Source: CAD feature listing. Evaluate the final solid. Frame: model axes, mm. Round coordinates to 2 decimals unless told otherwise and drop trailing zeros. Write each loop counter-clockwise with the first axis right and the second up, starting at its lowest first coordinate (ties: lowest second). Pieces come first, ordered by that corner, then holes. Notation, with made-up numbers: (35.25, 68.5) -> (44.25, 68.5) arc R17 cw to (44.25, 101.5) -> close; hole circle Ø2 at (25, 81). An arc over 180 degrees is marked (long way). Put each result on its own line as item: value.
```python
from build123d import *

# Parameters (mm, degrees)
F0_W           = 144
F0_H           = 20
F1_DEPTH       = 6
F3_D           = 6.7564
F3_DEPTH       = 16.51
F3_CSINK_D     = 13.4874
F3_CSINK_ANGLE = 82


with BuildPart() as f1:
    # F0 (on Top) → F1 (new body)
    with BuildSketch(Plane.XY):
        Rectangle(F0_W, F0_H)
    extrude(amount=F1_DEPTH)

    # F3
    with Locations(Plane.XY.offset(6)):
        with Locations((-34, 0), (36, 0)):
            CounterSinkHole(F3_D / 2, F3_CSINK_D / 2, depth=F3_DEPTH, counter_sink_angle=F3_CSINK_ANGLE)


solid = f1.part
```
Q1. Cut plane C-C on z = 4.45. Output: boundary loops of the cut face in (x, y).
Ans:
outline: (-72, -10) -> (72, -10) -> (72, 10) -> (-72, 10) -> close; hole circle Ø10.79 at (-34, 0); hole circle Ø10.79 at (36, 0)
Q2. Draft query along X for faces 1 (the flat face through (-1, 0, 6)), 2 (the conical face through (39.54, 0.16, 2.32)), 3 (the flat face through (72, 0, 3)). Return one class per face: +X half, -X half, draft (parallel to the pull), parting line (faces both ways), or undercut.
Ans:
face 1: draft
face 2: undercut
face 3: +X half
Q3. Cut plane B-B on y = 0. Output: boundary loops of the cut face in (x, z).
Ans:
outline: (-72, 0) -> (-37.38, 0) -> (-37.38, 2.13) -> (-40.74, 6) -> (-72, 6) -> close; (-30.62, 0) -> (32.62, 0) -> (32.62, 2.13) -> (29.26, 6) -> (-27.26, 6) -> (-30.62, 2.13) -> close; (39.38, 0) -> (72, 0) -> (72, 6) -> (42.74, 6) -> (39.38, 2.13) -> close
Q4. Material intervals for line 1 (X direction, y = 0, z = 0.5); line 2 (Y direction, x = -34, z = 0.55); line 3 (X direction, y = -1.75, z = 2.8), sorted ascending. Write a range as [from, to].
Ans:
line 1: x = [-72, -37.38], [-30.62, 32.62], [39.38, 72]
line 2: y = [-10, -3.38], [3.38, 10]
line 3: x = [-72, -37.55], [-30.45, 32.45], [39.55, 72]
Q5. Pin query (flat end, axial travel): pin 1 (9 mm diameter, centred on x = -34, y = 0, fed in from -Z); pin 2 (6 mm diameter, centred on x = 36, y = 0, fed in from -Z). Return the tip coordinate at first contact, or that it passes through.
Ans:
pin 1: stops at z = 0
pin 2: passes through
Q6. Cut plane A-A on x = -34. Output: boundary loops of the cut face in (y, z), and give its area (3 significant figures).
Ans:
outline: (-10, 0) -> (-3.38, 0) -> (-3.38, 2.13) -> (-6.74, 6) -> (-10, 6) -> close; (3.38, 0) -> (10, 0) -> (10, 6) -> (6.74, 6) -> (3.38, 2.13) -> close
area: 66.4 mm^2
